```python
from build123d import *

# Parameters (mm, degrees)
F0_W       = 20
F0_H       = 20
F0_R       = 3.15
F1_DEPTH   = 20
F2_W       = 6
F2_H       = 3
F2_W_2     = 3
F2_H_2     = 6
F3_DEPTH   = 10
F6_D       = 3.3
F6_ON_F5_D = 3.3
F7_R       = 1


with BuildPart() as f1:
    # F0 (on Front) → F1 (new body)
    with BuildSketch(Plane.XZ):
        Rectangle(F0_W, F0_H)
        Circle(F0_R, mode=Mode.SUBTRACT)
    extrude(amount=F1_DEPTH)

    # F2 (on face) → F3 (cut)
    with BuildSketch(Plane.XZ.offset(20)):
        with Locations((0, 6)):
            Rectangle(F2_W, F2_H)
        with Locations((-6, 0)):
            Rectangle(F2_W_2, F2_H_2)
        with Locations((6, 0)):
            Rectangle(F2_W_2, F2_H_2)
        with Locations((0, -6)):
            Rectangle(F2_W, F2_H)
    extrude(amount=-F3_DEPTH, mode=Mode.SUBTRACT)

    # F6 (through all)
    with Locations(Plane.XY.offset(10)):
        with Locations((0, -15)):
            Hole(F6_D / 2)

    # F6 on F5 (through all)
    with Locations(Plane(origin=(-10, 0, 0), x_dir=(0, -1, 0), z_dir=(-1, 0, 0))):
        with Locations((15, 0)):
            Hole(F6_ON_F5_D / 2)

    # F7
    f7_edges = [f1.edges().sort_by_distance(p)[0] for p in [
        (-10, -10, 10),
        (10, -10, 10),
        (-10, -10, -10),
        (10, -10, -10),
    ]]
    fillet(f7_edges, radius=F7_R)


solid = f1.part
```
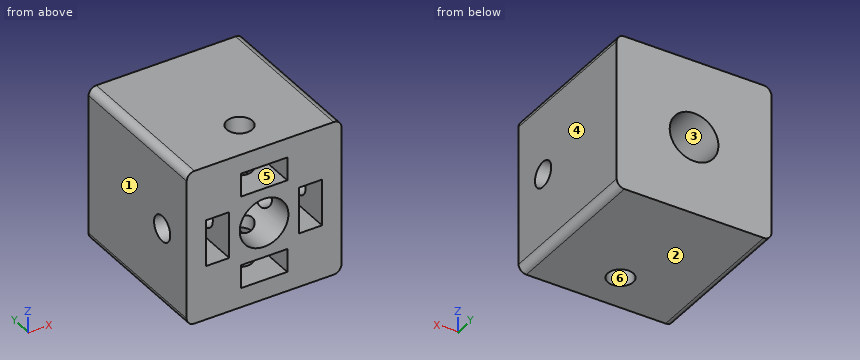
Input: part model. Units: mm. Frame: model coordinates. Face numbers are marked on the shaded views. A direction names the side the tool comes from. Coordinates: 2 decimals unless noted, no trailing zeros. Write each loop counter-clockwise with the first axis right and the second up, starting at its lowest first coordinate (ties: lowest second). Pieces come first, ordered by that corner, then holes.
1) Pin query (flat end, axial travel): pin 1 Ø1.5 at (x, z) = (0, -6.5) entering from -Y; pin 2 Ø5 at (x, z) = (4, -5.5) entering from +Y. Return the tip coordinate at first contact, or that it passes through.
2) Set-up query: the marked faces 5 and 6. Return all of +Z, -Z, +X, -X, +Y, -Y with unobstructed straight access to the full face (end or side cutting, diameter ignored); none if empty.
3) Section D-D on y = -6. Output: boundary loops of the cut face in (x, z), and give its area (3 significant figures).
4) Section A-A on y = -11. Output: boundary loops of the cut face in (x, z).
5) Material intervals for line 1 along X through (y, z) = (-10.75, -4.75); line 2 along Z through (x, y) = (3.7, -15); line 3 along Y through (x, z) = (0, 9.4), sorted ascending.
6) Section B-B on z = 0. State how many separate pieces and enclosed holes the cut face has, and give its area (3 significant figures).
7) Mould query, pull axis X, two halves, no side actions, for the marked faces 1, 2, 3 and 4. Classes: pulls with the +X half, pulls with the -X half, needs draft (parallel to the pull), parting line crosses it, or undercut.
Check result:
1. pin 1: stops at y = -10
1. pin 2: stops at y = 0
2. face 5: -Y
2. face 6: +Z, -Z
3. outline: (-10, -9) arc R1 ccw to (-9, -10) - (9, -10) arc R1 ccw to (10, -9) - (10, 9) arc R1 ccw to (9, 10) - (-9, 10) arc R1 ccw to (-10, 9) - close; hole circle Ø6.3 at (0, 0)
3. area: 368 mm2
4. outline: (-10, -9) arc R1 ccw to (-9, -10) - (9, -10) arc R1 ccw to (10, -9) - (10, 9) arc R1 ccw to (9, 10) - (-9, 10) arc R1 ccw to (-10, 9) - close; hole (-7.5, -3) - (-4.5, -3) - (-4.5, 3) - (-7.5, 3) - close; hole circle Ø6.3 at (0, 0); hole (-3, -7.5) - (3, -7.5) - (3, -4.5) - (-3, -4.5) - close; hole (-3, 4.5) - (3, 4.5) - (3, 7.5) - (-3, 7.5) - close; hole (4.5, -3) - (7.5, -3) - (7.5, 3) - (4.5, 3) - close
5. line 1: x = -10 to -3, 3 to 10
5. line 2: z = -10 to -1.65, 1.65 to 10
5. line 3: y = -20 to -16.65, -13.35 to 0
6. separate pieces: 6
6. enclosed holes: 0
6. area: 189 mm2
7. face 1: pulls with the -X half
7. face 2: needs draft
7. face 3: undercut
7. face 4: pulls with the +X half
